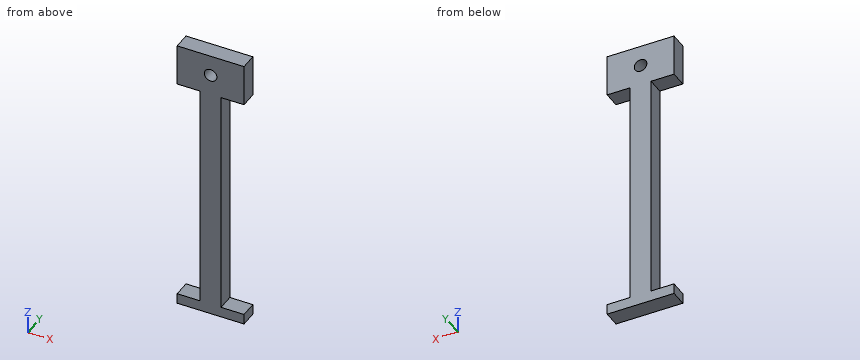
```python
from build123d import *

# Parameters (mm, degrees)
BOSS_EXTRUDE1_DEPTH = 4
SKETCH2_W           = 16
SKETCH2_H           = 4
BOSS_EXTRUDE2_DEPTH = 10
SKETCH3_R           = 1.5
CUT_EXTRUDE1_DEPTH  = 10


with BuildPart() as part:
    # Sketch1 → Boss-Extrude1 (new body)
    with BuildSketch(Plane(origin=(0, 0, 0), x_dir=(1, 0, 0), z_dir=(0, 1, 0))):
        Polygon((8, 57.5), (-8, 57.5), (-8, 55), (-2.5, 55), (-2.5, 0), (2.5, 0), (2.5, 55), (8, 55), align=None)
    extrude(amount=BOSS_EXTRUDE1_DEPTH)

    # Sketch2 → Boss-Extrude2 (add)
    with BuildSketch(Plane.XY):
        with Locations((0, 2)):
            Rectangle(SKETCH2_W, SKETCH2_H)
    extrude(amount=BOSS_EXTRUDE2_DEPTH)

    # Sketch3 → Cut-Extrude1 (cut)
    with BuildSketch(Plane(origin=(0, 4, 0), x_dir=(1, 0, 0), z_dir=(0, 1, 0))):
        with Locations((0, -5)):
            Circle(SKETCH3_R)
    extrude(amount=-CUT_EXTRUDE1_DEPTH, mode=Mode.SUBTRACT)


solid = part.part
```
Geometry: final body of the model. Coordinates: model frame, mm. Coordinates: 2 decimals unless noted, no trailing zeros. Order: outer loops, then holes, each group sorted by start corner. A loop starts at its lowest first (then second) coordinate and runs counter-clockwise, first axis right, second up. Notation, with made-up numbers: (23.5, -34.75) -> (60.5, -34.75) arc R27 cw to (60.5, -11.75) -> close; hole circle Ø2 at (-8.75, -26.75). An arc over 180 degrees is marked (long way). Write each question's results on one line, items separated by ' | '. Start each with the question number.
1) Cut plane C-C, the plane z = 5. Output: boundary loops of the cut face in (x, y), and give its area (3 significant figures).
2) Cut plane A-A, the plane x = -3.5. Output: boundary loops of the cut face in (y, z), and give its area (3 significant figures).
3) First-contact query: pin 1 (1.5 mm diameter, centred on y = 1.5, z = -39.5, fed in from -X); pin 2 (2 mm diameter, centred on y = 1.5, z = -21.5, fed in from +X). Flat tips, straight axial feed; report the tip coordinate or a pass-through.
4) Cut plane B-B, the plane y = 1.15. Output: boundary loops of the cut face in (x, z), and give its area (3 significant figures).
5) Cut plane D-D, the plane z = -5. Output: boundary loops of the cut face in (x, y), and give its area (3 significant figures).
6) Material intervals for line 1 along Z through (x, y) = (0, 1.4); line 2 along Z through (x, y) = (-4, 2.2); line 3 along X through (y, z) = (1.5, 5), sorted ascending.
Checks:
1) outline: (-8, 0) -> (-1.5, 0) -> (-1.5, 4) -> (-8, 4) -> close; (1.5, 0) -> (8, 0) -> (8, 4) -> (1.5, 4) -> close | area: 52.0 mm^2
2) outline: (0, -57.5) -> (4, -57.5) -> (4, -55) -> (0, -55) -> close; (0, 0) -> (4, 0) -> (4, 10) -> (0, 10) -> close | area: 50.0 mm^2
3) pin 1: x = -2.5 | pin 2: x = 2.5
4) outline: (-8, -57.5) -> (8, -57.5) -> (8, -55) -> (2.5, -55) -> (2.5, 0) -> (8, 0) -> (8, 10) -> (-8, 10) -> (-8, 0) -> (-2.5, 0) -> (-2.5, -55) -> (-8, -55) -> close; hole circle Ø3 at (0, 5) | area: 468 mm^2
5) outline: (-2.5, 0) -> (2.5, 0) -> (2.5, 4) -> (-2.5, 4) -> close | area: 20.0 mm^2
6) line 1: -57.5 to 3.5, 6.5 to 10 | line 2: -57.5 to -55, 0 to 10 | line 3: -8 to -1.5, 1.5 to 8
